Design review of the part built by this model. Coordinates are the model's own, in mm. A direction names the side the tool comes from. Round coordinates to 2 decimals unless told otherwise and drop trailing zeros. Loops run counter-clockwise (first coordinate to the right, second up) from the corner with the lowest first, then second, coordinate; pieces in that order, holes last. Notation, with made-up numbers: (14, 49) - (29, 49) arc R18 ccw to (29, 73) - close; hole circle Ø4 at (54, 12.25). An arc over 180 degrees is marked (long way). Return JSON: item names as keys, results as strings. Group by question number.
(1) For faces 1 (the flat face through (-371.475, -9, -10)), 2 (the cylindrical face through (429.39, 11.732, -4.864)), 3 (the flat face through (5.2, 7.24, 12.32)), list the 3-axis set-ups (+Z, -Z, +X, -X, +Y, -Y) from which the entire face can be reached by the end or side of a thin tool; tool diameter is ignored.
(2) Wall thickness on L1, parallel to X at y = 12.5, z = 2; L2, parallel to X at y = -5.25, z = -13 (3 decimals); L3, parallel to Z at x = 310.5, y = -6.5 (3 decimals): over which ranges is each line inside the solid? List them lowest first. Write a range as [from, to].
(3) We need section A-A, the plane x = -246. Write out the cut boundary in (y, z), and give its area (3 significant figures).
(4) Clearance check with flat-ended pins moving along their axes: pin 1 (8 mm diameter, centred on x = 383.5, y = -5.5, fed in from +Z); pin 2 (1.5 mm diameter, centred on y = -10, z = -10.5, fed in from +X) (3 decimals); pin 3 (8 mm diameter, centred on x = -268.5, y = -11, fed in from +Z). State where each tip first meets the part, or that it passes through.
(5) We need section B-B, the plane y = 5.25. Give the number of separate pieces and of enclosed holes in the cut face, and give its area (3 significant figures).
from build123d import *

# Parameters (mm, degrees)
PAD_DEPTH     = 371.475
SKETCH001_R   = 12.7
PAD001_DEPTH  = 117.475
SKETCH002_R   = 12.7
PAD002_DEPTH  = 15.875
SKETCH003_R   = 2.38125
SKETCH003_R_2 = 1.5875
SKETCH003_R_3 = 3.96875
SKETCH003_R_4 = 3.175
POCKET_DEPTH  = 50.8


with BuildPart() as part:
    # Sketch → Pad (new body, symmetric)
    with BuildSketch(Plane.YZ):
        Polygon((14.2875, -8.248892), (14.2875, 8.248892), (0, 16.497784), (-14.2875, 8.248892), (-14.2875, -8.248892), (0, -16.497784), align=None)
    extrude(amount=PAD_DEPTH, both=True)

    # Sketch001 (on Face8 of Pad) → Pad001 (join)
    with BuildSketch(Plane.YZ.offset(371.475)):
        Circle(SKETCH001_R)
    extrude(amount=PAD001_DEPTH)

    # Sketch002 (on Face4 of Pad001) → Pad002 (join)
    with BuildSketch(Plane(origin=(-371.475, 0, 0), x_dir=(0, 1, 0), z_dir=(-1, 0, 0))):
        Circle(SKETCH002_R)
    extrude(amount=PAD002_DEPTH)

    # Sketch003 (on Face8 of Pad002) → Pocket (cut)
    with BuildSketch(Plane(origin=(0, -14.2875, 0), x_dir=(0, 0, -1), z_dir=(0, -1, 0))):
        Circle(SKETCH003_R)
        with Locations((0, 368.3)):
            Circle(SKETCH003_R)
        with Locations((0, -368.3)):
            Circle(SKETCH003_R)
        with Locations((0, 400.05)):
            Circle(SKETCH003_R_2)
        with Locations((0, 479.425)):
            Circle(SKETCH003_R_3)
        with Locations((0, 431.8)):
            Circle(SKETCH003_R_4)
    extrude(amount=-POCKET_DEPTH, mode=Mode.SUBTRACT)


solid = part.part
Solutions:
{
 "1": {"face 1": "-X", "face 2": "+X", "face 3": "+Z, +X, -X, +Y"},
 "2": {"L1": "[-387.35, -369.59], [-367.01, -1.29], [1.29, 367.01], [369.59, 429.33], [434.27, 476], [482.85, 488.95]", "L2": "[-371.475, 371.475]", "L3": "[-12.745, 12.745]"},
 "3": {"outline": "(-14.29, -8.25) - (0, -16.5) - (14.29, -8.25) - (14.29, 8.25) - (0, 16.5) - (-14.29, 8.25) - close", "area": "707 mm^2"},
 "4": {"pin 1": "z = 12.61", "pin 2": "x = 371.475", "pin 3": "z = 12.46"},
 "5": {"separate pieces": "1", "enclosed holes": "6", "area": "23,000 mm^2"}
}
